Autodesk Inventor part; units mm, degrees
ref_plane "EAGF_XY" through (0, 0, 18) normal (0, 0, -1) x (1, 0, 0)
ref_plane "EAGF_YZ" through (0, 0, 18) normal (1, 0, 0) x (0, -1, 0)
ref_plane "EAGF_ZX" through (0, 0, 18) normal (0, -1, 0) x (0, 0, -1)
sketch "Sketch_1" plane through (0, 0, 0) normal (1, 0, 0) x (0, 1, 0)
  line L0 (0, -384) -> (0, 18)
  line L1 (0, 18) -> (4.8, 18)
  line L2 (4.8, 18) -> (5, 17.8)
  line L3 (5, 17.8) -> (5, 13.2)
  arc A0 (5, 13.2) -> (5.4, 12.8) centre (5.4, 13.2) ccw
  line L4 (5.4, 12.8) -> (8.035, 12.8)
  line L5 (8.035, 12.8) -> (8.335, 12.5)
  line L6 (8.335, 12.5) -> (8.335, 3.1)
  arc A1 (8.335, 3.1) -> (8.635, 2.8) centre (8.635, 3.1) ccw
  line L7 (8.635, 2.8) -> (8.635, -374)
  line L8 (8.635, -374) -> (16.6667, -374)
  line L9 (16.6667, -374) -> (16.6667, -384)
  line L10 (16.6667, -384) -> (0, -384)
  line L11 (0, -384) -> (0, 18)
revolve "Revolution1" add sketch "Sketch_1" angle 360 about axis through (0, 0, -384) along (0, 0, -1)
sketch "Sketch_3" plane through (0, 0, 0) normal (1, 0, 0) x (0, 1, 0)
  line L0 (0, 18) -> (0, 34)
  line L1 (0, 34) -> (3.233, 34)
  line L2 (3.233, 34) -> (4, 33.233)
  line L3 (4, 33.233) -> (4, 20.8321)
  line L4 (4, 20.8321) -> (3.0804, 19.2392)
  arc A0 (3.0804, 19.2392) -> (3, 18.9392) centre (3.6, 18.9392) ccw
  line L5 (3, 18.9392) -> (3, 18.6)
  arc A1 (3, 18.6) -> (3.6, 18) centre (3.6, 18.6) ccw
  line L6 (3.6, 18) -> (0, 18)
  line L7 (0, 18) -> (0, 34)
revolve "Revolution2" add sketch "Sketch_3" angle 360 about axis through (0, 0, 18) along (0, 0, -1)
thread "Thread1"
sketch "Sketch_2" plane through (0, 0, 18) normal (0, 0, 1) x (1, 0, 0)
  line L0 (-6.5, 7) -> (-6.5, -5)
  line L1 (-6.5, -5) -> (-4.5, -5)
  line L2 (-4.5, -5) -> (-4.5, 5)
  line L3 (-4.5, 5) -> (4.5, 5)
  line L4 (4.5, 5) -> (4.5, -5)
  line L5 (4.5, -5) -> (6.5, -5)
  line L6 (6.5, -5) -> (6.5, 7)
  line L7 (6.5, 7) -> (-6.5, 7)
extrude "Extrusion1" cut sketch "Sketch_2" against normal blind 4.2
ref_plane "EAGF_XY" through (0, 0, 18) normal (0, 0, -1) x (1, 0, 0)
ref_plane "EAGF_YZ" through (0, 0, 18) normal (1, 0, 0) x (0, -1, 0)
ref_plane "EAGF_ZX" through (0, 0, 18) normal (0, -1, 0) x (0, 0, -1)
ref_plane "EPCO_KS_XY" through (0, 0, 0) normal (0, 0, -1) x (1, 0, 0)
ref_plane "EPCO_KS_YZ" through (0, 0, 0) normal (1, 0, 0) x (0, -1, 0)
ref_plane "EPCO_KS_ZX" through (0, 0, 0) normal (0, -1, 0) x (0, 0, -1)
ref_plane "NUT_XY" through (0, 0, 26) normal (0, 0, -1) x (1, 0, 0)
ref_plane "NUT_YZ" through (0, 0, 26) normal (1, 0, 0) x (0, -1, 0)
ref_plane "NUT_ZX" through (0, 0, 26) normal (0, -1, 0) x (0, 0, -1)
properties part number "1470874 EPCO-25-300_k---(1_0)"
Geometry check sheet. Reference: the model listing, model coordinates, mm. A direction names the side the tool comes from. Coordinates: 2 decimals unless noted, no trailing zeros. Order: outer loops, then holes, each group sorted by start corner. A loop starts at its lowest first (then second) coordinate and runs counter-clockwise, first axis right, second up. Notation, with made-up numbers: M 39,-27.5 L 77,-27.5 A10 ccw 77,-13.5 Z; hole C 48,16.25 d3. An arc over 180 degrees is marked long. One line per question, with ' | ' between items. Start each with the question number.
Item 1: Set-up check for faces 4 (the cylindrical face through (-3.905, -0.867, 26.946)), 5 (the cylindrical face through (-16.27, -3.61, -379.07)): record each of +Z, -Z, +X, -X, +Y, -Y from which the full face is reachable in a straight line by a thin tool's end or side.
Item 2: Gauge pin test, flat ends, axial feed: pin 1 (3.5 mm diameter, centred on y = -0.5, z = 16.5, fed in from +X); pin 2 (6 mm diameter, centred on x = 0.5, z = -171.5, fed in from +Y) (3 decimals); pin 3 (0.6 mm diameter, centred on x = 5, y = 0, fed in from +Z). Record the tip position at first contact, or that the pin passes through.
Item 3: Draft check along Z on faces 1 (the flat face through (0, 0, 34)), 2 (the flat face through (0, 0, -384)), 3 (the flat face through (3.1, -2.2, 18)). Enter one of: pulls with the +Z half, pulls with the -Z half, needs draft (parallel to the pull), parting line crosses it, or undercut.
Item 4: Material ranges on L1, parallel to Z at x = -11, y = 1.5; L2, parallel to Y at x = -7, z = -42; L3, parallel to Z at x = 4, y = 5.5, recorded low to high. Write a range as [from, to].
Item 5: Cross-section at A-A on z = -57.5. Enter the section's corners in (x, y) (3 decimals).
Findings:
1) face 4: +Z | face 5: +Z, -Z
2) pin 1: stops at x = 4.5 | pin 2: stops at y = 8.635 | pin 3: stops at z = 13.8
3) face 1: pulls with the +Z half | face 2: pulls with the -Z half | face 3: undercut
4) L1: z = [-384, -374] | L2: y = [-5.06, 5.06] | L3: z = [-384, 12.8]
5) outline: C 0,0 d17.27
